Design review of the part built by this model. Coordinates are the model's own, in mm. A direction names the side the tool comes from. Give positions to 0.01 mm unless a question says otherwise; leave off trailing zeros. Write each loop counter-clockwise with the first axis right and the second up, starting at its lowest first coordinate (ties: lowest second). Pieces come first, ordered by that corner, then holes. Notation, with made-up numbers: (52.5, 66) -> (56.5, 66) arc R32 cw to (56.5, 105) -> close; hole circle Ø7 at (16, 33.25). An arc over 180 degrees is marked (long way). Answer as a JSON object with one key per item and string values.
```python
from build123d import *

# Parameters (mm, degrees)
BASE_FLANGE1_DEPTH       = 177.8
SKETCH2_R                = 2.7051
CUT_EXTRUDE1_0213_DEPTH  = 7.62
SKETCH3_R                = 2.3114
CUT_EXTRUDE2_0_182_DEPTH = 7.62
SKETCH4_R                = 2.3114
CUT_EXTRUDE4_0_182_DEPTH = 7.62
SKETCH5_R                = 2.7051
CUT_EXTRUDE3_0_213_DEPTH = 7.62
FILLET1_R                = 6.35


# Sheet-metal steps are written as plain solids
with BuildPart() as part:
    # Sketch1 → Base-Flange1 (new body)
    with BuildSketch(Plane.XY):
        with BuildLine():
            Line((-139.7, 266.7), (-139.7, 248.649497326))
            ThreePointArc((-139.7, 248.649497326), (-139.516321312, 247.726082204), (-138.993248663, 246.943248663))
            Line((-138.993248663, 246.943248663), (-70.088063608, 178.038063608))
            ThreePointArc((-70.088063608, 178.038063608), (-69.911870716, 177.77437231), (-69.85, 177.463327217))
            Line((-69.85, 177.463327217), (-69.85, 2.413))
            ThreePointArc((-69.85, 2.413), (-69.143248663, 0.706751337), (-67.437, 0))
            Line((-67.437, 0), (-50.8, 0))
            Line((-50.8, 0), (-50.8, 1.6002))
            Line((-50.8, 1.6002), (-67.437, 1.6002))
            ThreePointArc((-67.437, 1.6002), (-68.011736392, 1.838263608), (-68.2498, 2.413))
            Line((-68.2498, 2.413), (-68.2498, 177.463327217))
            ThreePointArc((-68.2498, 177.463327216), (-68.433478688, 178.386742339), (-68.956551337, 179.16957588))
            Line((-68.956551337, 179.16957588), (-137.861736392, 248.074760934))
            ThreePointArc((-137.861736392, 248.074760934), (-138.037929284, 248.338452232), (-138.0998, 248.649497326))
            Line((-138.0998, 248.649497326), (-138.0998, 266.7))
            Line((-138.0998, 266.7), (-139.7, 266.7))
        make_face()
    extrude(amount=BASE_FLANGE1_DEPTH)

    # Sketch2 → Cut-Extrude1 .0213 (cut)
    with BuildSketch(Plane.XZ):
        with Locations(Location((-58.7248, 19.05, 0), (0, 0, 270))):
            Circle(SKETCH2_R)
        with Locations(Location((-58.7248, 88.9, 0), (0, 0, 270))):
            Circle(SKETCH2_R)
        with Locations(Location((-58.7248, 158.75, 0), (0, 0, 270))):
            Circle(SKETCH2_R)
    extrude(amount=-CUT_EXTRUDE1_0213_DEPTH, mode=Mode.SUBTRACT)

    # Sketch3 → Cut-Extrude2 0.182 (cut)
    with BuildSketch(Plane(origin=(-68.2498, 0, 0), x_dir=(0, 0, -1), z_dir=(1, 0, 0))):
        with Locations(Location((-168.275, 139.7, 0), (0, 0, 90))):
            Circle(SKETCH3_R)
        with Locations(Location((-168.275, 38.1, 0), (0, 0, 90))):
            Circle(SKETCH3_R)
        with Locations(Location((-9.525, 139.7, 0), (0, 0, 90))):
            Circle(SKETCH3_R)
        with Locations(Location((-9.525, 38.1, 0), (0, 0, 90))):
            Circle(SKETCH3_R)
    extrude(amount=-CUT_EXTRUDE2_0_182_DEPTH, mode=Mode.SUBTRACT)

    # Sketch4 → Cut-Extrude4 0.182 (cut)
    with BuildSketch(Plane(origin=(55.106512271, 55.106512271, 0), x_dir=(0, 0, -1), z_dir=(0.7071067811865511, 0.707106781186544, 0))):
        with Locations(Location((-168.275, 225.914994361, 0), (0, 0, 90))):
            Circle(SKETCH4_R)
        with Locations(Location((-9.525, 225.914994361, 0), (0, 0, 90))):
            Circle(SKETCH4_R)
    extrude(amount=-CUT_EXTRUDE4_0_182_DEPTH, mode=Mode.SUBTRACT)

    # Sketch5 → Cut-Extrude3 0.213 (cut)
    with BuildSketch(Plane(origin=(-138.0998, 0, 0), x_dir=(0, 0, -1), z_dir=(1, 0, 0))):
        with Locations((-158.75, 257.175)):
            Circle(SKETCH5_R)
        with Locations((-88.9, 257.175)):
            Circle(SKETCH5_R)
        with Locations((-19.05, 257.175)):
            Circle(SKETCH5_R)
    extrude(amount=-CUT_EXTRUDE3_0_213_DEPTH, mode=Mode.SUBTRACT)

    # Fillet1
    fillet1_edges = [part.edges().sort_by_distance(p)[0] for p in [
        (-50.8, 0.8001, 0),
        (-138.8999, 266.7, 0),
        (-50.8, 0.8001, 177.8),
        (-138.8999, 266.7, 177.8),
    ]]
    fillet(fillet1_edges, radius=FILLET1_R)


solid = part.part
```
(1) Clearance check with flat-ended pins moving along their axes: pin 1 (1 mm diameter, centred on x = -92, z = 130, fed in from -Y); pin 2 (3 mm diameter, centred on x = -91, z = 32, fed in from -Y); pin 3 (1 mm diameter, centred on x = -103, z = 105, fed in from -Y); pin 4 (4.5 mm diameter, centred on x = -58.72, z = 88.9, fed in from +Y). State where each tip first meets the part, or that it passes through.
Here are the results:
{"pin 1": "stops at y = 199.45", "pin 2": "stops at y = 197.45", "pin 3": "stops at y = 210.45", "pin 4": "passes through"}
(2) The part is to be moulded in two halves that separate along X. For faces 3 (the flat face through (-138.1, 262, 88)), 4 (the cylindrical face through (-138.91, 264.89, 1.91)), 5 (the cylindrical face through (-57.91, 0.79, 86.32)), 6 (the cylindrical face through (-57.91, 0.79, 156.17)), say which applies: +X half, -X half, draft (parallel to the pull), parting line (faces both ways), or undercut.
Here are the results:
{"face 3": "+X half", "face 4": "draft", "face 5": "undercut", "face 6": "undercut"}
(3) For faces 1 (the flat face through (-139.7, 260, 88)), 2 (the flat face through (-68.25, 89, 88)), list the 3-axis set-ups (+Z, -Z, +X, -X, +Y, -Y) from which the entire face can be reached by the end or side of a thin tool; tool diameter is ignored.
Here are the results:
{"face 1": "+Z, -Z, -X, +Y, -Y", "face 2": "+Z, -Z, +X, +Y"}
(4) We need section A-A, the plane z = 158.75. State the section outline as (x, y) points, then the cut area to 3 significant figures.
Here are the results:
{"outline": "(-139.7, 248.65) arc R2.41 ccw to (-138.99, 246.94) -> (-70.09, 178.04) arc R0.81 cw to (-69.85, 177.46) -> (-69.85, 2.41) arc R2.41 ccw to (-67.44, 0) -> (-61.43, 0) -> (-61.43, 1.6) -> (-67.44, 1.6) arc R0.81 cw to (-68.25, 2.41) -> (-68.25, 177.46) arc R2.41 ccw to (-68.96, 179.17) -> (-137.86, 248.07) arc R0.81 cw to (-138.1, 248.65) -> (-138.1, 254.47) -> (-139.7, 254.47) -> close; (-139.7, 259.88) -> (-138.1, 259.88) -> (-138.1, 266.7) -> (-139.7, 266.7) -> close; (-56.02, 0) -> (-50.8, 0) -> (-50.8, 1.6) -> (-56.02, 1.6) -> close", "area": "482 mm²"}
(5) For line 1 along Z through (x, y) = (-69.2, 139.7); line 2 along Y through (x, z) = (-60, 66.5); line 3 along X through (y, z) = (80.5, 51), list the stretches that pass through material, from the lowest coordinate up.
Here are the results:
{"line 1": "z = 0 to 7.21, 11.84 to 165.96, 170.59 to 177.8", "line 2": "y = 0 to 1.6", "line 3": "x = -69.85 to -68.25"}
(6) We need section D-D, the plane x = -131. State the section outline as (y, z) points, then the cut area to 3 significant figures.
Here are the results:
{"outline": "(238.95, 0) -> (241.21, 0) -> (241.21, 177.8) -> (238.95, 177.8) -> close", "area": "402 mm²"}
(7) We need section B-B, the plane z = 98. State the section outline as (x, y) points, then the cut area to 3 significant figures.
Here are the results:
{"outline": "(-139.7, 248.65) arc R2.41 ccw to (-138.99, 246.94) -> (-70.09, 178.04) arc R0.81 cw to (-69.85, 177.46) -> (-69.85, 2.41) arc R2.41 ccw to (-67.44, 0) -> (-50.8, 0) -> (-50.8, 1.6) -> (-67.44, 1.6) arc R0.81 cw to (-68.25, 2.41) -> (-68.25, 177.46) arc R2.41 ccw to (-68.96, 179.17) -> (-137.86, 248.07) arc R0.81 cw to (-138.1, 248.65) -> (-138.1, 266.7) -> (-139.7, 266.7) -> close", "area": "500 mm²"}
(8) We need section C-C, the plane y = 33. State the section outline as (x, z) points, then the cut area to 3 significant figures.
Here are the results:
{"outline": "(-69.85, 0) -> (-68.25, 0) -> (-68.25, 177.8) -> (-69.85, 177.8) -> close", "area": "285 mm²"}
